The model under review builds one solid part; all positions refer to its coordinate system, in mm. Round coordinates to 2 decimals unless told otherwise and drop trailing zeros. Order: outer loops, then holes, each group sorted by start corner. A loop starts at its lowest first (then second) coordinate and runs counter-clockwise, first axis right, second up. Notation, with made-up numbers: (-9.5, 52) -> (-4.5, 52) arc R28 ccw to (-4.5, 70) -> close; hole circle Ø6 at (-25.75, -32.75). An arc over 180 degrees is marked (long way). Use a Markdown table: item, result. Add a question column.
Autodesk Inventor part; units mm, degrees
ref_plane "YZ Plane" through (0, 0, 0) normal (1, 0, 0) x (0, 1, 0)
ref_plane "XZ Plane" through (0, 0, 0) normal (0, 1, 0) x (-1, 0, 0)
ref_plane "XY Plane" through (0, 0, 0) normal (0, 0, 1) x (1, 0, 0)
sketch "Sketch1" plane through (0, 0, 0) normal (1, 0, 0) x (0, 1, 0)
  arc A0 (1.9313, -2.4249) -> (-1.9054, -2.4453) centre (0, 0) ccw
  circle A1 centre (0, 0) radius 6
  line L0 (-3.1, 0) -> (-3.1, 2) construction
  line L1 (-1.9054, -2.4453) -> (1.9313, -2.4249)
  line L2 (0, 1) -> (-20, 1)
  line L3 (-20, 1) -> (-20, -1)
  line L4 (-20, -1) -> (0, -1)
  line L5 (0, -1) -> (0, 1)
  point P0 (-5.9161, -1)
  point P1 (-5.9161, 1)
  dimension "d0" = 6.2
  dimension "d1" = 12
  dimension "d2" = 2
  dimension "d5" = 1
  dimension "d6" = 2
  dimension "d7" = 20
extrude "Extrusion1" add sketch "Sketch1" along normal blind 2 contours A0 L2 A1 L4 L1 | A0 L4 A1 L2 | A1 L4 L3 L2
equation "\"d6\" = 2 * d5"
properties part number "tarcza krańcówek"
Q1. Draft analysis for pull direction Z (two halves, no side actions). For faces 1 (the face through (1, -13, -1)), 2 (the face through (2, -4, 0)), 3 (the face through (1, -13, 1)), 4 (the face through (1, -0.1, 3.1)), state which applies: released by +Z, released by -Z, zero draft, split by the parting line, or undercut.
Q2. For pin 1 (3.5 mm diameter, centred on y = 0, z = 0, fed in from +X); pin 2 (0.6 mm diameter, centred on x = 1, y = -12, fed in from +Z); pin 3 (1 mm diameter, centred on x = 1.5, z = 1, fed in from +Y); pin 4 (1 mm diameter, centred on x = 1, y = -6, fed in from -Z), all flat-tipped, find the tip position at first contact; note any pin that passes through.
Q3. Add section D-D, the plane y = -7.75. Give the boundary of the cut face in (x, z).
Q4. Add section B-B, the plane y = 0.25. Give the boundary of the cut face in (x, z).
Q5. Add section C-C, the plane x = 0.35. Give the boundary of the cut face in (y, z), then the cut area to 3 significant figures.
Q6. To check wall thickness, follow line 1 along Y through (x, z) = (0.1, 0); line 2 along Z through (x, y) = (1, -8.25); line 3 along Y through (x, z) = (0.35, 2.5). State the ranges of each line that lie inside material, in increasing order.
Q7. Add section A-A, the plane z = 0. Give the boundary of the cut face in (x, y), then the cut area to 3 significant figures.
Return value:
| question | item | result |
|---|---|---|
| 1 | face 1 | released by -Z |
| 1 | face 2 | zero draft |
| 1 | face 3 | released by +Z |
| 1 | face 4 | undercut |
| 2 | pin 1 | through |
| 2 | pin 2 | z = 1 |
| 2 | pin 3 | y = 5.98 |
| 2 | pin 4 | z = -2.4 |
| 3 | outline | (0, -1) -> (2, -1) -> (2, 1) -> (0, 1) -> close |
| 4 | outline | (0, -5.99) -> (2, -5.99) -> (2, -2.43) -> (0, -2.43) -> close; (0, 3.09) -> (2, 3.09) -> (2, 5.99) -> (0, 5.99) -> close |
| 5 | outline | (-20, -1) -> (-5.92, -1) arc R6 ccw (long way) to (-5.92, 1) -> (-20, 1) -> close; hole (-1.91, -2.45) -> (1.93, -2.42) arc R3.1 ccw (long way) to start |
| 5 | area | 113 mm² |
| 6 | line 1 | -20 to -3.1, 3.1 to 6 |
| 6 | line 2 | -1 to 1 |
| 6 | line 3 | -5.45 to -1.83, 1.83 to 5.45 |
| 7 | outline | (0, -20) -> (2, -20) -> (2, -3.1) -> (0, -3.1) -> close; (0, 3.1) -> (2, 3.1) -> (2, 6) -> (0, 6) -> close |
| 7 | area | 39.6 mm² |
